Build history of the part. All positions in model axes, mm. Face numbers are marked on the shaded views. A direction names the side the tool comes from. Coordinates: 2 decimals unless noted, no trailing zeros. Loops run counter-clockwise (first coordinate to the right, second up) from the corner with the lowest first, then second, coordinate; pieces in that order, holes last. Notation, with made-up numbers: M -13.75,84.25 L 31.25,84.25 A18 ccw 31.25,100.25 Z; hole C -5.5,45.5 d4. An arc over 180 degrees is marked long. Write each question's results on one line, items separated by ' | '. Start each with the question number.
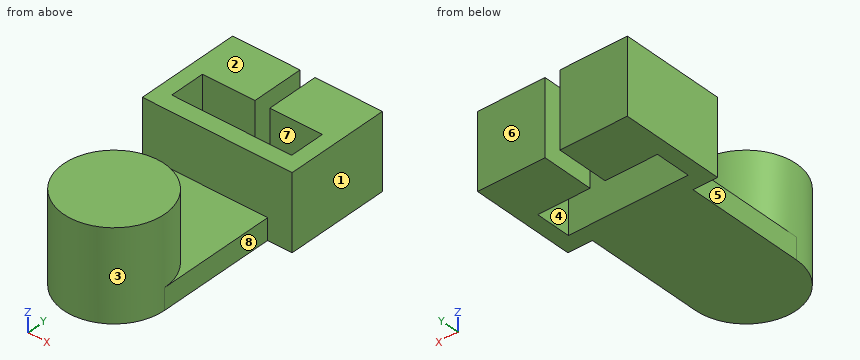
from build123d import *

# Parameters (mm, degrees)
SKETCH1_R           = 10.6807
BOSS_EXTRUDE1_DEPTH = 19.05
SKETCH2_W           = 21.3614
SKETCH2_H           = 25.4
BOSS_EXTRUDE2_DEPTH = 4.5212
BOSS_EXTRUDE3_DEPTH = 3.556
SKETCH4_W           = 15.875
SKETCH4_H           = 22.225
BOSS_EXTRUDE4_DEPTH = 3.175
SKETCH5_W           = 15.875
SKETCH5_H           = 22.225
BOSS_EXTRUDE5_DEPTH = 3.175
SKETCH7_W           = 15.875
SKETCH7_H           = 11.1125
BOSS_EXTRUDE6_DEPTH = 11.1125
SKETCH8_W           = 15.875
SKETCH8_H           = 11.1125
BOSS_EXTRUDE7_DEPTH = 11.1125


with BuildPart() as part:
    # Sketch1 → Boss-Extrude1 (new body)
    with BuildSketch(Plane.XY):
        with Locations(Location((0, 0, 0), (0, 0, 180))):
            Circle(SKETCH1_R)
    extrude(amount=BOSS_EXTRUDE1_DEPTH)

    # Sketch2 → Boss-Extrude2 (add)
    with BuildSketch(Plane(origin=(0, 0, 0), x_dir=(-1, 0, 0), z_dir=(0, 0, -1))):
        with Locations((0, 12.7)):
            Rectangle(SKETCH2_W, SKETCH2_H)
    extrude(amount=-BOSS_EXTRUDE2_DEPTH)

    # Sketch3 → Boss-Extrude3 (add)
    with BuildSketch(Plane(origin=(0, 25.4, 0), x_dir=(1, 0, 0), z_dir=(0, 1, 0))):
        Polygon((0, 0), (12.7, 0), (12.7, -15.875), (-12.7, -15.875), (-12.7, 0), align=None)
    extrude(amount=BOSS_EXTRUDE3_DEPTH)

    # Sketch4 → Boss-Extrude4 (add)
    with BuildSketch(Plane(origin=(12.7, 0, 0), x_dir=(0, 0, -1), z_dir=(1, 0, 0))):
        with Locations((-7.9375, 36.5125)):
            Rectangle(SKETCH4_W, SKETCH4_H)
    extrude(amount=BOSS_EXTRUDE4_DEPTH)

    # Sketch5 → Boss-Extrude5 (add)
    with BuildSketch(Plane.ZY.offset(12.7)):
        with Locations((7.9375, 36.5125)):
            Rectangle(SKETCH5_W, SKETCH5_H)
    extrude(amount=BOSS_EXTRUDE5_DEPTH)

    # Sketch7 → Boss-Extrude6 (add)
    with BuildSketch(Plane(origin=(-12.7, 0, 0), x_dir=(0, 0, -1), z_dir=(1, 0, 0))):
        with Locations((-7.9375, 42.06875)):
            Rectangle(SKETCH7_W, SKETCH7_H)
    extrude(amount=BOSS_EXTRUDE6_DEPTH)

    # Sketch8 → Boss-Extrude7 (add)
    with BuildSketch(Plane.ZY.offset(-12.7)):
        with Locations((7.9375, 42.06875)):
            Rectangle(SKETCH8_W, SKETCH8_H)
    extrude(amount=BOSS_EXTRUDE7_DEPTH)


solid = part.part
1. Which spindle directions (+Z, -Z, +X, -X, +Y, -Y) get a long thin tool onto all of the face, cutting with end or side? Do the marked faces 1, 2, 3, 4 and 5. Say none if no direction does.
2. Wall check: line 1 along X through (y, z) = (45, 4) (1 decimal); line 2 along Y through (x, z) = (-11, 7) (1 decimal); line 3 along X through (y, z) = (31, 14.5) (3 decimals). Give the ranges that are in metal, low to high.
3. Band-saw the part on C-C, the plane x = 0. List the corners of the cut face in (y, z) (3 decimals), plus the area to 3 significant figures.
4. Band-saw the part on D-D, the plane z = 3.5. List the corners of the cut face in (x, y) (1 decimal).
5. Pin check, flat tips, straight feed: pin 1 (8 mm diameter, centred on y = -2.5, z = 6.5, fed in from -X); pin 2 (8 mm diameter, centred on y = 10.5, z = 17, fed in from +X); pin 3 (3.5 mm diameter, centred on y = 9.5, z = 3.5, fed in from +X). Stop position of each tip, or through.
6. Band-saw the part on A-A, the plane z = 13.5. List the corners of the cut face in (x, y) (1 decimal).
7. Mould opens along X. For the marked faces 6, 7 and 8 say: +X half, -X half, draft (parallel to the pull), parting line (faces both ways), or undercut.
Checked values:
1) face 1: +Z, -Z, +X, +Y, -Y | face 2: +Z, +X, -X, +Y | face 3: +Z | face 4: +Z, -Z | face 5: +Z, -Z, -X, -Y
2) line 1: -15.9 to -1.6, 1.6 to 15.9 | line 2: 25.4 to 29, 36.5 to 47.6 | line 3: -15.875 to -12.7, 12.7 to 15.875
3) outline: M -10.681,0 L 28.956,0 L 28.956,15.875 L 25.4,15.875 L 25.4,4.521 L 10.681,4.521 L 10.681,19.05 L -10.681,19.05 Z | area: 530 mm²
4) outline: M -15.9,25.4 L -10.7,25.4 L -10.7,0 A10.7 ccw 10.7,0 L 10.7,25.4 L 15.9,25.4 L 15.9,47.6 L 1.6,47.6 L 1.6,36.5 L 12.7,36.5 L 12.7,29 L -12.7,29 L -12.7,36.5 L -1.6,36.5 L -1.6,47.6 L -15.9,47.6 Z
5) pin 1: x = -10.68 | pin 2: x = 8.48 | pin 3: x = 10.68
6) outline: M -15.9,25.4 L 15.9,25.4 L 15.9,47.6 L 1.6,47.6 L 1.6,36.5 L 12.7,36.5 L 12.7,29 L -12.7,29 L -12.7,36.5 L -1.6,36.5 L -1.6,47.6 L -15.9,47.6 Z; C 0,0 d21.4
7) face 6: draft | face 7: undercut | face 8: +X half
